from build123d import *

# Parameters (mm, degrees)
MODEL_W            = 113
MODEL_H            = 52.9
MODEL_R            = 0.8
MODEL_R_2          = 1.59995
MODEL_W_2          = 1.6
MODEL_H_2          = 1.6
BOSS_EXTRU_1_DEPTH = 1.6


with BuildPart() as part:
    # Model → Boss.-Extru.1 (new body)
    with BuildSketch(Plane.XY):
        with Locations((56.5, 26.45)):
            Rectangle(MODEL_W, MODEL_H)
        with Locations((52.3, 50.5)):
            Circle(MODEL_R, mode=Mode.SUBTRACT)
        with Locations((49.76, 50.5)):
            Circle(MODEL_R, mode=Mode.SUBTRACT)
        with Locations((47.22, 50.5)):
            Circle(MODEL_R, mode=Mode.SUBTRACT)
        with Locations((44.68, 50.5)):
            Circle(MODEL_R, mode=Mode.SUBTRACT)
        with Locations((42.14, 50.5)):
            Circle(MODEL_R, mode=Mode.SUBTRACT)
        with Locations((39.6, 50.5)):
            Circle(MODEL_R, mode=Mode.SUBTRACT)
        with Locations((37.06, 50.5)):
            Circle(MODEL_R, mode=Mode.SUBTRACT)
        with Locations((34.52, 50.5)):
            Circle(MODEL_R, mode=Mode.SUBTRACT)
        with Locations((30.46, 50.5)):
            Circle(MODEL_R, mode=Mode.SUBTRACT)
        with Locations((27.92, 50.5)):
            Circle(MODEL_R, mode=Mode.SUBTRACT)
        with Locations((25.38, 50.5)):
            Circle(MODEL_R, mode=Mode.SUBTRACT)
        with Locations((22.84, 50.5)):
            Circle(MODEL_R, mode=Mode.SUBTRACT)
        with Locations((20.3, 50.5)):
            Circle(MODEL_R, mode=Mode.SUBTRACT)
        with Locations((17.76, 50.5)):
            Circle(MODEL_R, mode=Mode.SUBTRACT)
        with Locations((15.22, 50.5)):
            Circle(MODEL_R, mode=Mode.SUBTRACT)
        with Locations((12.68, 50.5)):
            Circle(MODEL_R, mode=Mode.SUBTRACT)
        with Locations((10.14, 50.5)):
            Circle(MODEL_R, mode=Mode.SUBTRACT)
        with Locations((7.6, 50.5)):
            Circle(MODEL_R, mode=Mode.SUBTRACT)
        with Locations((19.28, 2.24)):
            Circle(MODEL_R, mode=Mode.SUBTRACT)
        with Locations((21.82, 2.24)):
            Circle(MODEL_R, mode=Mode.SUBTRACT)
        with Locations((24.36, 2.24)):
            Circle(MODEL_R, mode=Mode.SUBTRACT)
        with Locations((26.9, 2.24)):
            Circle(MODEL_R, mode=Mode.SUBTRACT)
        with Locations((29.44, 2.24)):
            Circle(MODEL_R, mode=Mode.SUBTRACT)
        with Locations((31.98, 2.24)):
            Circle(MODEL_R, mode=Mode.SUBTRACT)
        with Locations((34.52, 2.24)):
            Circle(MODEL_R, mode=Mode.SUBTRACT)
        with Locations((39.6, 2.24)):
            Circle(MODEL_R, mode=Mode.SUBTRACT)
        with Locations((42.14, 2.24)):
            Circle(MODEL_R, mode=Mode.SUBTRACT)
        with Locations((44.68, 2.24)):
            Circle(MODEL_R, mode=Mode.SUBTRACT)
        with Locations((47.22, 2.24)):
            Circle(MODEL_R, mode=Mode.SUBTRACT)
        with Locations((49.76, 2.24)):
            Circle(MODEL_R, mode=Mode.SUBTRACT)
        with Locations((52.3, 2.24)):
            Circle(MODEL_R, mode=Mode.SUBTRACT)
        with Locations((105, 3)):
            Circle(MODEL_R_2, mode=Mode.SUBTRACT)
        with Locations((105, 50)):
            Circle(MODEL_R_2, mode=Mode.SUBTRACT)
        with Locations((3, 50)):
            Circle(MODEL_R_2, mode=Mode.SUBTRACT)
        with Locations((3, 3)):
            Circle(MODEL_R_2, mode=Mode.SUBTRACT)
        with Locations((16.74, 2.24)):
            Rectangle(MODEL_W_2, MODEL_H_2, mode=Mode.SUBTRACT)
    extrude(amount=BOSS_EXTRU_1_DEPTH)


solid = part.part
Work out the finished part from the listing and answer in its coordinate system (mm). Round coordinates to 2 decimals unless told otherwise and drop trailing zeros. One line per item, written item: value.
Q1. Flat-ended cylindrical pins translate along their axes: pin 1 (1 mm diameter, centred on x = 39.6, y = 50.5, fed in from -Z); pin 2 (1.5 mm diameter, centred on x = 57, y = 22.5, fed in from -Z). Find the tip coordinate at first contact, or state that the pin passes through.
Derived:
pin 1: through
pin 2: z = 0
Q2. Determine the mould class of faces 1 (the face through (56, 27, 0)), 2 (the face through (1.82, 4.08, 0.79)) for opening direction Y: released by +Y, released by -Y, zero draft, split by the parting line, or undercut.
Derived:
face 1: zero draft
face 2: undercut
Q3. Find section A-A on z = 0.5. Give the number of separate pieces and of enclosed holes in the cut face, then the cut area to 3 significant figures.
Derived:
separate pieces: 1
enclosed holes: 36
area: 5,880 mm²
Q4. Straight lines are drawn through the part: line 1 (Y direction, x = 3, z = 0.9); line 2 (Y direction, x = 39.6, z = 0.55); line 3 (Y direction, x = 21.82, z = 1.1). For each, find the intervals that lie inside material, in ascending order.
Derived:
line 1: 0 to 1.4, 4.6 to 48.4, 51.6 to 52.9
line 2: 0 to 1.44, 3.04 to 49.7, 51.3 to 52.9
line 3: 0 to 1.44, 3.04 to 52.9
